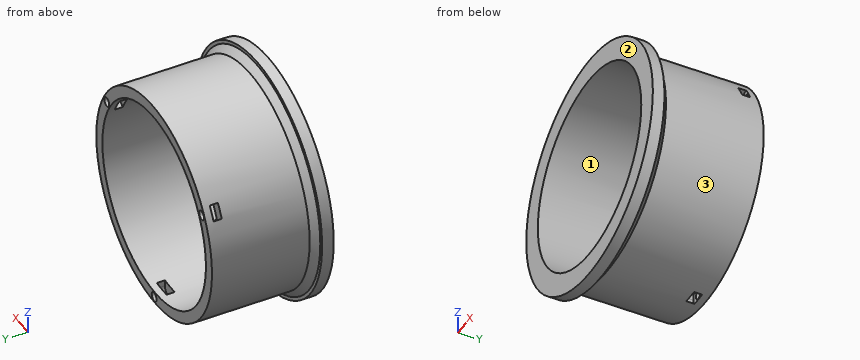
Autodesk Inventor part; units mm, degrees
ref_plane "Work Plane1" through (0, 45, 0) normal (0, 1, 0) x (1, 0, 0)
ref_plane "YZ Plane" through (0, 0, 0) normal (1, 0, 0) x (0, 1, 0)
ref_plane "XZ Plane" through (0, 0, 0) normal (0, 1, 0) x (-1, 0, 0)
sketch "Sketch1" plane through (0, 0, 0) normal (0, 0, 1) x (1, 0, 0)
  line L0 (42.5, 0) -> (42.5, 50)
  line L1 (0, -10) -> (0, 60)
  line L2 (42.5, 0) -> (52, 0)
  line L3 (52, 0) -> (52, 5)
  line L4 (52, 5) -> (50.5, 5)
  line L5 (47.5, 8) -> (47.5, 50)
  line L6 (-10.4, 0) -> (62.4, 0)
  line L7 (50.5, 5) -> (47.5, 8)
  line L8 (42.5, 50) -> (47.5, 50)
  point P0 (0, 0)
  point P1 (47.5, 5)
  point P2 (45, 50)
  dimension "d1" = 5
  dimension "d6" = 3
  dimension "d7" = 3
  dimension "d8" = 50
  dimension "d30" = 9.5
  dimension "d31" = 45
  dimension "d32" = 5
revolve "Revolution1" add sketch "Sketch1" angle 360 about axis through (0, -10, 0) along (0, 1, 0)
ref_plane "Work Plane1" through (0, 45, 0) normal (0, 1, 0) x (1, 0, 0)
sketch "Sketch2" plane through (0, 45, 0) normal (0, 1, 0) x (1, 0, 0)
  arc A0 (-3.996, 44.8222) -> (3.996, 44.8222) centre (0, 0) ccw
  arc A1 (3.996, 44.8222) -> (-3.996, 44.8222) centre (0, 45) ccw
  circle A2 centre (0, 0) radius 42.5
  line L0 (4, 45) -> (4, 41.0512)
  line L1 (4, 41.0512) -> (-4, 41.0512)
  line L2 (-4, 41.0512) -> (-4, 45)
  point P0 (0, 44.7796)
  point P1 (-4, 44.8219)
  point P2 (-4, 42.3113)
  point P3 (4, 42.3113)
  point P4 (4, 44.8219)
  dimension "d11" = 90
  dimension "d12" = 8
extrude "Nut Seat" cut sketch "Sketch2" along normal mid plane 3.5 contours A1 A0 L0 A2 L2 | A0 L2 A1 | A0 A1 L0 | L2 L1 L0 A2 | A2 L0 L1 L2
sketch "Sketch3" plane through (0, 50, 0) normal (0, 1, 0) x (1, 0, 0)
  line L0 (0, 72.8) -> (0, -72.8)
  point P0 (0, 0)
  point P1 (0, 45)
  dimension "d26" = 45
hole "Hole1" at (0, 50, -45) direction (0, -1, 0) diameter 4 depth 6.75
pattern_circular "Circular Pattern1" count 3 over 360 about axis through (0, -10, 0) along (0, 1, 0) of "Hole1"
pattern_circular "Circular Pattern2" count 3 over 360 about axis through (0, 25, 0) along (0, 1, 0) of "Nut Seat"
properties part number "Center Cylinder"
CAD build for the part. Positions are in the model's coordinates, mm. Face numbers are marked on the shaded views. Give positions to 0.01 mm unless a question says otherwise; leave off trailing zeros. Loops run counter-clockwise (first coordinate to the right, second up) from the corner with the lowest first, then second, coordinate; pieces in that order, holes last. Notation, with made-up numbers: M 63,71.25 L 97,71.25 A20 cw 97,94.25 Z; hole C 37,-26.5 d6. An arc over 180 degrees is marked long. Answer in a Markdown table with one row per item. Add a question column.
Item 1: Band-saw the part on A-A on z = 0. Give the cut face in (x, y).
Item 2: Band-saw the part on B-B on x = 0. Give the cut face in (y, z).
Item 3: Band-saw the part on C-C on y = 13. Give the cut face in (x, z).
Item 4: Mould opens along Z. For the marked faces 1, 2 and 3 say: +Z half, -Z half, draft (parallel to the pull), parting line (faces both ways), or undercut.
Item 5: Drop flat-ended pins along their axis: P1, Ø3, axis at x = -11.5, y = 31.5, coming from the -Z side; P2, Ø5, axis at x = -8.5, y = 33.5, coming from the +Z side; P3, Ø8, axis at y = 6.5, z = -10.5, coming from the +X side. Give the stop position or say it passes through.
Item 6: Probe probe 1 along X at (y, z) = (48.8, 22.5); probe 2 along Z at (x, y) = (0, 29); probe 3 along X at (y, z) = (23.5, 1). List the from-to ranges inside material, lowest first.
Reply:
| question | item | result |
|---|---|---|
| 1 | outline | M -52,0 L -42.5,0 L -42.5,50 L -47.5,50 L -47.5,8 L -50.5,5 L -52,5 Z; M 42.5,0 L 52,0 L 52,5 L 50.5,5 L 47.5,8 L 47.5,50 L 42.5,50 Z |
| 2 | outline | M 0,-52 L 5,-52 L 5,-50.5 L 8,-47.5 L 43.25,-47.5 L 43.25,-42.5 L 0,-42.5 Z; M 0,42.5 L 50,42.5 L 50,47.5 L 8,47.5 L 5,50.5 L 5,52 L 0,52 Z; M 46.75,-47.5 L 50,-47.5 L 50,-47 L 46.75,-47 Z; M 46.75,-43 L 50,-43 L 50,-42.5 L 46.75,-42.5 Z |
| 3 | outline | C 0,0 d95; hole C 0,0 d85 |
| 4 | face 1 | undercut |
| 4 | face 2 | draft |
| 4 | face 3 | parting line |
| 5 | P1 | stops at z = -46.44 |
| 5 | P2 | stops at z = 47.12 |
| 5 | P3 | stops at x = 51.55 |
| 6 | probe 1 | x = -41.83 to -40.97, -36.97 to -36.06, 36.06 to 36.97, 40.97 to 41.83 |
| 6 | probe 2 | z = -47.5 to -42.5, 42.5 to 47.5 |
| 6 | probe 3 | x = -47.49 to -42.49, 42.49 to 47.49 |
